Check sheet for the modelled part. Datum: model origin and axes. Units: mm. A direction names the side the tool comes from. Round coordinates to 2 decimals unless told otherwise and drop trailing zeros. Order: outer loops, then holes, each group sorted by start corner. A loop starts at its lowest first (then second) coordinate and runs counter-clockwise, first axis right, second up.
Q1. Mould release check, pull along X, two halves, no side actions. Record for faces 1 (the flat face through (0, 7, 25.4)), 2 (the flat face through (0, 88, 0)), 3 (the flat face through (6.35, 88, 14)): +X half, -X half, draft (parallel to the pull), parting line (faces both ways), or undercut.
Q2. Cross-section at D-D on y = 57.5. Record the cut outline in (x, z) (3 decimals), then the cut area to 3 significant figures.
Q3. Cross-section at C-C on y = 158. Record the cut outline in (x, z) (3 decimals), then the cut area to 3 significant figures.
Q4. Cross-section at B-B on z = 14. Record the cut outline in (x, y) (3 decimals), then the cut area to 3 significant figures.
Q5. Set-up check for faces 4 (the flat face through (0, 171, 25.4)), 5 (the flat face through (-3.175, 88, 15)), 6 (the cylindrical face through (4.78, 89.93, 24.85)): record each of +Z, -Z, +X, -X, +Y, -Y from which the full face is reachable in a straight line by a thin tool's end or side.
Q6. Scan lines: probe 1 along Y at (x, z) = (-2.25, 4.5); probe 2 along X at (y, z) = (134, 15) (3 decimals); probe 3 along Z at (x, y) = (-0.25, 90) (3 decimals). Record each from-to range of solid material in increasing order.
Q7. Cross-section at A-A on x = 0.25. Record the cut outline in (y, z) (3 decimals), then the cut area to 3 significant figures.
Q8. Depth check by flat-ended pin: P1, Ø3, axis at x = -0.5, y = 7, coming from the +Z side; P2, Ø7, axis at x = 1.5, y = 172.5, coming from the +Z side; P3, Ø5, axis at x = 0.5, y = 123.5, coming from the +Z side (3 decimals). Enter the tip coordinate at first touch or a pass-through.
from build123d import *

# Parameters (mm, degrees)
F0_W        = 152.4
F0_H        = 3.175
F1_DEPTH    = 6.35
F2_DEPTH    = 3.175
F3_T1_DEPTH = 86.5404436654
F3_T3_DEPTH = 86.5404436654


# Not quite as in the source:
# - a fillet or chamfer that OpenCascade refuses, or shapes differently, is made with other operations: its cross-section is extruded or revolved along the edge and cut away or added


with BuildPart() as f1:
    # F0 (on Right) → F1 (new body, symmetric)
    with BuildSketch(Plane.YZ):
        with Locations((88.9, 1.5875)):
            Rectangle(F0_W, F0_H)
        Polygon((0, 25.4), (0, 0), (12.7, 0), (12.7, 3.175), (12.7, 25.4), align=None)
        Polygon((165.1, 3.175), (165.1, 0), (177.8, 0), (177.8, 25.4), (165.1, 25.4), align=None)
        with BuildLine():
            Line((0, 38.1), (0, 25.4))
            Line((0, 25.4), (12.7, 25.4))
            Line((12.7, 25.4), (12.7, 3.175))
            Line((12.7, 3.175), (165.1, 3.175))
            Line((165.1, 3.175), (165.1, 25.4))
            Line((165.1, 25.4), (177.8, 25.4))
            Line((177.8, 25.4), (177.8, 38.1))
            ThreePointArc((177.8, 38.1), (88.9, 24.8473031945), (0, 38.1))
        make_face()
    extrude(amount=F1_DEPTH, both=True)

    # F0 (on Right) → F2 (cut, symmetric)
    with BuildSketch(Plane.YZ):
        with BuildLine():
            Line((0, 38.1), (0, 25.4))
            Line((0, 25.4), (12.7, 25.4))
            Line((12.7, 25.4), (12.7, 3.175))
            Line((12.7, 3.175), (165.1, 3.175))
            Line((165.1, 3.175), (165.1, 25.4))
            Line((165.1, 25.4), (177.8, 25.4))
            Line((177.8, 25.4), (177.8, 38.1))
            ThreePointArc((177.8, 38.1), (88.9, 24.8473031945), (0, 38.1))
        make_face()
    extrude(amount=F2_DEPTH, both=True, mode=Mode.SUBTRACT)

    # F3: fillet of radius 12.7 on 4 edges, made by hand

    # F3_s2 → F3_t1 (cut)
    with BuildSketch(Plane.YZ.offset(-48.0327218327)):
        with BuildLine():
            ThreePointArc((0, 21.4269112669), (4.8711942162, 31.4269012669), (15.748, 33.755726944))
            ThreePointArc((15.748, 33.755726944), (7.8448900248, 35.8223397437), (0, 38.1))
            Line((0, 38.1), (0, 21.4269112669))
        make_face()
        with BuildLine():
            ThreePointArc((177.8, 21.4269112669), (172.9288057838, 31.4269012669), (162.052, 33.755726944))
            ThreePointArc((162.052, 33.755726944), (169.9551099752, 35.8223397437), (177.8, 38.1))
            Line((177.8, 38.1), (177.8, 21.4269112669))
        make_face()
    extrude(amount=F3_T1_DEPTH, mode=Mode.SUBTRACT)

    # F3_s4 → F3_t3 (cut)
    with BuildSketch(Plane.YZ.offset(-38.5077218327)):
        with BuildLine():
            ThreePointArc((0, 21.4269112669), (4.8711942162, 31.4269012669), (15.748, 33.755726944))
            ThreePointArc((15.748, 33.755726944), (7.8448900248, 35.8223397437), (0, 38.1))
            Line((0, 38.1), (0, 21.4269112669))
        make_face()
        with BuildLine():
            ThreePointArc((177.8, 21.4269112669), (172.9288057838, 31.4269012669), (162.052, 33.755726944))
            ThreePointArc((162.052, 33.755726944), (169.9551099752, 35.8223397437), (177.8, 38.1))
            Line((177.8, 38.1), (177.8, 21.4269112669))
        make_face()
    extrude(amount=F3_T3_DEPTH, mode=Mode.SUBTRACT)


solid = f1.part
Results found:
1. face 1: undercut
1. face 2: draft
1. face 3: +X half
2. outline: (-6.35, 0) - (6.35, 0) - (6.35, 26.469) - (3.175, 26.469) - (3.175, 3.175) - (-3.175, 3.175) - (-3.175, 26.469) - (-6.35, 26.469) - close
2. area: 188 mm2
3. outline: (-6.35, 0) - (6.35, 0) - (6.35, 32.783) - (3.175, 32.783) - (3.175, 3.175) - (-3.175, 3.175) - (-3.175, 32.783) - (-6.35, 32.783) - close
3. area: 228 mm2
4. outline: (-6.35, 0) - (6.35, 0) - (6.35, 177.8) - (-6.35, 177.8) - close; hole (-3.175, 12.7) - (3.175, 12.7) - (3.175, 165.1) - (-3.175, 165.1) - close
4. area: 1,290 mm2
5. face 4: +Z, +Y, -Y
5. face 5: +Z
5. face 6: +Z, +X, -X
6. probe 1: y = 0 to 12.7, 165.1 to 177.8
6. probe 2: x = -6.35 to -3.175, 3.175 to 6.35
6. probe 3: z = 0 to 3.175
7. outline: (0, 0) - (177.8, 0) - (177.8, 21.427) arc R12.7 ccw to (177.163, 25.4) - (165.1, 25.4) - (165.1, 3.175) - (12.7, 3.175) - (12.7, 25.4) - (0.637, 25.4) arc R12.7 ccw to (0, 21.427) - close
7. area: 1,130 mm2
8. P1: stops at z = 25.4
8. P2: stops at z = 33.37
8. P3: stops at z = 3.175
